from build123d import *

# Parameters (mm, degrees)
F0_R           = 35
F0_R_2         = 16
F1_DEPTH       = 15
F2_SIZE        = 1
F4_D           = 6
F4_CSINK_D     = 10
F4_CSINK_ANGLE = 90


with BuildPart() as f1:
    # F0 (on Right) → F1 (new body)
    with BuildSketch(Plane.YZ):
        Circle(F0_R)
        Circle(F0_R_2, mode=Mode.SUBTRACT)
    extrude(amount=F1_DEPTH)

    # F2
    f2_edges = [f1.edges().sort_by_distance(p)[0] for p in [
        (15, -35, 0),
        (0, -35, 0),
    ]]
    chamfer(f2_edges, length=F2_SIZE)

    # F4 (through all)
    with Locations(Plane.YZ.offset(15)):
        with Locations((0, 25), (-25, 0), (25, 0), (0, -25)):
            CounterSinkHole(F4_D / 2, F4_CSINK_D / 2, counter_sink_angle=F4_CSINK_ANGLE)


solid = f1.part
The model under review builds one solid part; all positions refer to its coordinate system, in mm. Round coordinates to 2 decimals unless told otherwise and drop trailing zeros. Loops run counter-clockwise (first coordinate to the right, second up) from the corner with the lowest first, then second, coordinate; pieces in that order, holes last. Notation, with made-up numbers: (26.5, 50.25) -> (43.5, 50.25) arc R14 cw to (43.5, 62.25) -> close; hole circle Ø9 at (16, 20). An arc over 180 degrees is marked (long way). Write item = value, one per line. Start each with the question number.
Item 1: Take a section at A-A on z = 0. Give the boundary of the cut face in (x, y).
Item 2: Mouldability with a two-part tool opening along Y and no side actions: class faces 1 (the cylindrical face through (6.41, 0.65, -27.93)), 2 (the cylindrical face through (6.41, 0.65, 22.07)), 3 (the flat face through (0, 15, -7)), 4 (the cylindrical face through (7, -28, -21)) as released by +Y, released by -Y, zero draft, split by the parting line, or undercut.
Item 3: Insertion check: pin 1 (7 mm diameter, centred on y = 25, z = 0, fed in from +X); pin 2 (8 mm diameter, centred on x = 11, y = 1, fed in from -Z); pin 3 (5 mm diameter, centred on x = 2, z = 10, fed in from -Y); pin 4 (5 mm diameter, centred on y = 0, z = -25, fed in from -X). Each pin has a flat end and moves straight along its axis. Give the tip position at first contact, or say it passes through.
Item 4: Take a section at C-C on x = 8. Give the boundary of the cut face in (y, z).
Item 5: To check wall thickness, follow L1, parallel to Z at x = 3, y = 0; L2, parallel to Z at x = 3.75, y = 18; L3, parallel to Y at x = 9.25, z = 25. State the ranges of each line that lie inside material, in increasing order.
Result:
q1.outline = (0, -34) -> (1, -35) -> (14, -35) -> (15, -34) -> (15, -30) -> (13, -28) -> (0, -28) -> close; (0, -22) -> (13, -22) -> (15, -20) -> (15, -16) -> (0, -16) -> close; (0, 16) -> (15, 16) -> (15, 20) -> (13, 22) -> (0, 22) -> close; (0, 28) -> (13, 28) -> (15, 30) -> (15, 34) -> (14, 35) -> (1, 35) -> (0, 34) -> close
q2.face_1 = undercut
q2.face_2 = undercut
q2.face_3 = zero draft
q2.face_4 = split by the parting line
q3.pin_1 = 13.5
q3.pin_2 = -35
q3.pin_3 = -34.19
q3.pin_4 = through
q4.outline = circle Ø70 at (0, 0); hole circle Ø6 at (-25, 0); hole circle Ø32 at (0, 0); hole circle Ø6 at (0, -25); hole circle Ø6 at (0, 25); hole circle Ø6 at (25, 0)
q5.L1 = -35 to -28, -22 to -16, 16 to 22, 28 to 35
q5.L2 = -30.02 to 30.02
q5.L3 = -24.49 to -3, 3 to 24.49
